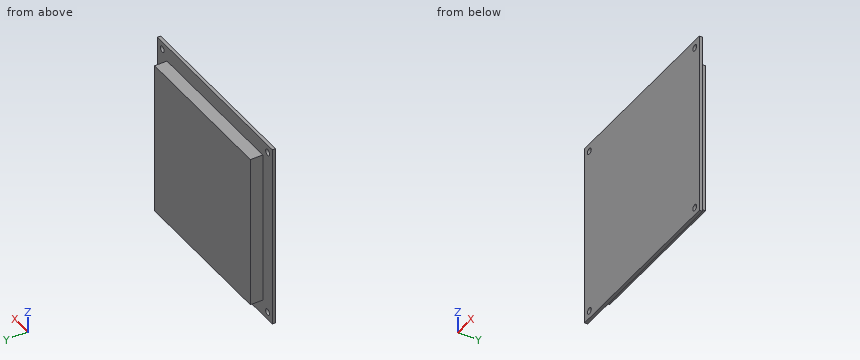
from build123d import *

# Parameters (mm, degrees)
SKETCH1_W           = 152.4
SKETCH1_H           = 152.4
BOSS_EXTRUDE1_DEPTH = 2.54
SKETCH9_R           = 2.54
CUT_EXTRUDE5_DEPTH  = 3.54
SKETCH10_W          = 127
SKETCH10_H          = 127
BOSS_EXTRUDE2_DEPTH = 10.16


with BuildPart() as part:
    # Sketch1 → Boss-Extrude1 (new body)
    with BuildSketch(Plane(origin=(0, 0, 0), x_dir=(1, 0, 0), z_dir=(0, 1, 0))):
        Rectangle(SKETCH1_W, SKETCH1_H)
    extrude(amount=-BOSS_EXTRUDE1_DEPTH)

    # Sketch9 → Cut-Extrude5 (cut, through all)
    with BuildSketch(Plane(origin=(0, 0, 0), x_dir=(1, 0, 0), z_dir=(0, 1, 0))):
        with Locations((-69.85, -69.85)):
            Circle(SKETCH9_R)
        with Locations((69.85, -69.85)):
            Circle(SKETCH9_R)
        with Locations((69.85, 69.85)):
            Circle(SKETCH9_R)
        with Locations((-69.85, 69.85)):
            Circle(SKETCH9_R)
    extrude(amount=-CUT_EXTRUDE5_DEPTH, mode=Mode.SUBTRACT)

    # Sketch10 → Boss-Extrude2 (add)
    with BuildSketch(Plane(origin=(0, 0, 0), x_dir=(1, 0, 0), z_dir=(0, 1, 0))):
        Rectangle(SKETCH10_W, SKETCH10_H)
    extrude(amount=BOSS_EXTRUDE2_DEPTH)


solid = part.part
The model under review builds one solid part; all positions refer to its coordinate system, in mm. Round coordinates to 2 decimals unless told otherwise and drop trailing zeros. Order: outer loops, then holes, each group sorted by start corner. A loop starts at its lowest first (then second) coordinate and runs counter-clockwise, first axis right, second up. Notation, with made-up numbers: (46.5, 11) -> (104.5, 11) arc R36 cw to (104.5, 48) -> close; hole circle Ø6 at (-7.5, -27). An arc over 180 degrees is marked (long way). Use CSV: the item, a comma, the result in double quotes. Start each with the question number.
(1) Consider section D-D on x = 45. Write out the cut boundary in (y, z).
(2) Wall thickness on probe 1 along Z at (x, y) = (-69.85, -0.7); probe 2 along X at (y, z) = (9.75, -50.5): over which ranges is each line inside the solid? List them lowest first. Write a range as from..to.
(3) Consider section A-A on x = -69.85. Write out the cut boundary in (y, z), and give its area (3 significant figures).
(4) Consider section B-B on z = -69.85. Write out the cut boundary in (x, y).
(5) Insertion check: pin 1 (3 mm diameter, centred on y = 3, z = 7.5, fed in from +X); pin 2 (6.5 mm diameter, centred on x = 69.85, z = 69.85, fed in from +Y); pin 3 (2 mm diameter, centred on x = 24.5, y = 8, fed in from -Z). Each pin has a flat end and moves straight along its axis. Give the tip position at first contact, or say it passes through.
(6) Consider section C-C on z = -16. Write out the cut boundary in (x, y).
Responses:
1,outline,"(-2.54, -76.2) -> (0, -76.2) -> (0, -63.5) -> (10.16, -63.5) -> (10.16, 63.5) -> (0, 63.5) -> (0, 76.2) -> (-2.54, 76.2) -> close"
2,probe 1,"-76.2..-72.39, -67.31..67.31, 72.39..76.2"
2,probe 2,"-63.5..63.5"
3,outline,"(-2.54, -76.2) -> (0, -76.2) -> (0, -72.39) -> (-2.54, -72.39) -> close; (-2.54, -67.31) -> (0, -67.31) -> (0, 67.31) -> (-2.54, 67.31) -> close; (-2.54, 72.39) -> (0, 72.39) -> (0, 76.2) -> (-2.54, 76.2) -> close"
3,area,"361 mm²"
4,outline,"(-76.2, -2.54) -> (-72.39, -2.54) -> (-72.39, 0) -> (-76.2, 0) -> close; (-67.31, -2.54) -> (67.31, -2.54) -> (67.31, 0) -> (-67.31, 0) -> close; (72.39, -2.54) -> (76.2, -2.54) -> (76.2, 0) -> (72.39, 0) -> close"
5,pin 1,"x = 63.5"
5,pin 2,"y = 0"
5,pin 3,"z = -63.5"
6,outline,"(-76.2, -2.54) -> (76.2, -2.54) -> (76.2, 0) -> (63.5, 0) -> (63.5, 10.16) -> (-63.5, 10.16) -> (-63.5, 0) -> (-76.2, 0) -> close"
